```python
from build123d import *

# Parameters (mm, degrees)
EXTRUDE_1_DEPTH             = 5
SKETCH_2_R                  = 1.6
CUT_EXTRUDE_1_DEPTH         = 5
PATTERN_LINEAR_1_COUNT      = 2
PATTERN_LINEAR_1_PITCH      = 58
PATTERN_LINEAR_1_COUNT_DIR2 = 2
PATTERN_LINEAR_1_PITCH_DIR2 = 49
SKETCH_3_R                  = 2.6
CUT_EXTRUDE_2_DEPTH         = 10
PATTERN_LINEAR_2_COUNT      = 2
PATTERN_LINEAR_2_PITCH      = 33
PATTERN_LINEAR_2_COUNT_DIR2 = 2
PATTERN_LINEAR_2_PITCH_DIR2 = 33
SKETCH_4_R                  = 1.65
CUT_EXTRUDE_4_DEPTH         = 10


with BuildPart() as part:
    # Эскиз1 → Бобышка-Вытянуть1 (new body)
    with BuildSketch(Plane(origin=(0, 0, 0), x_dir=(1, 0, 0), z_dir=(0, 1, 0))):
        Polygon((0, 0), (170, 0), (170, 60), (110, 190), (60, 190), (0, 60), align=None)
    extrude(amount=EXTRUDE_1_DEPTH)

    # Эскиз2 → Вырез-Вытянуть1 (cut)
    with BuildSketch(Plane(origin=(0, 5, 0), x_dir=(1, 0, 0), z_dir=(0, 1, 0))):
        with Locations(Location((60.5, 20, 0), (0, 0, 270))):
            Circle(SKETCH_2_R)
    cut_extrude_1 = extrude(amount=-CUT_EXTRUDE_1_DEPTH, mode=Mode.SUBTRACT)

    # Линейный массив1: Cut-Extrude 1 2 × 2
    with Locations(*[(j * PATTERN_LINEAR_1_PITCH_DIR2, 0, -i * PATTERN_LINEAR_1_PITCH) for i in range(PATTERN_LINEAR_1_COUNT) for j in range(PATTERN_LINEAR_1_COUNT_DIR2) if (i, j) != (0, 0)]):
        add(cut_extrude_1, mode=Mode.SUBTRACT)

    # Эскиз3 → Вырез-Вытянуть2 (cut)
    with BuildSketch(Plane(origin=(0, 5, 0), x_dir=(1, 0, 0), z_dir=(0, 1, 0))):
        with Locations(Location((101.5, 180, 0), (0, 0, 270))):
            Circle(SKETCH_3_R)
    cut_extrude_2 = extrude(amount=-CUT_EXTRUDE_2_DEPTH, mode=Mode.SUBTRACT)

    # Линейный массив2: Cut-Extrude 2 2 × 2
    with Locations(*[(-i * PATTERN_LINEAR_2_PITCH, 0, j * PATTERN_LINEAR_2_PITCH_DIR2) for i in range(PATTERN_LINEAR_2_COUNT) for j in range(PATTERN_LINEAR_2_COUNT_DIR2) if (i, j) != (0, 0)]):
        add(cut_extrude_2, mode=Mode.SUBTRACT)

    # Эскиз4 → Вырез-Вытянуть4 (cut)
    with BuildSketch(Plane(origin=(0, 5, 0), x_dir=(1, 0, 0), z_dir=(0, 1, 0))):
        with Locations(Location((23.75, 8.999743724, 0), (0, 0, 270))):
            Circle(SKETCH_4_R)
        with Locations(Location((23.75, 20.999743724, 0), (0, 0, 270))):
            Circle(SKETCH_4_R)
        with Locations(Location((146.25, 20.999743724, 0), (0, 0, 270))):
            Circle(SKETCH_4_R)
        with Locations(Location((146.25, 8.999743724, 0), (0, 0, 270))):
            Circle(SKETCH_4_R)
        with Locations(Location((45.274277733, 101.419560045, 0), (0, 0, 270))):
            Circle(SKETCH_4_R)
        with Locations(Location((40.245579603, 90.524047431, 0), (0, 0, 270))):
            Circle(SKETCH_4_R)
        with Locations(Location((126.821084869, 96.879607741, 0), (0, 0, 270))):
            Circle(SKETCH_4_R)
        with Locations(Location((131.849782999, 85.984095127, 0), (0, 0, 270))):
            Circle(SKETCH_4_R)
    extrude(amount=-CUT_EXTRUDE_4_DEPTH, mode=Mode.SUBTRACT)


solid = part.part
```
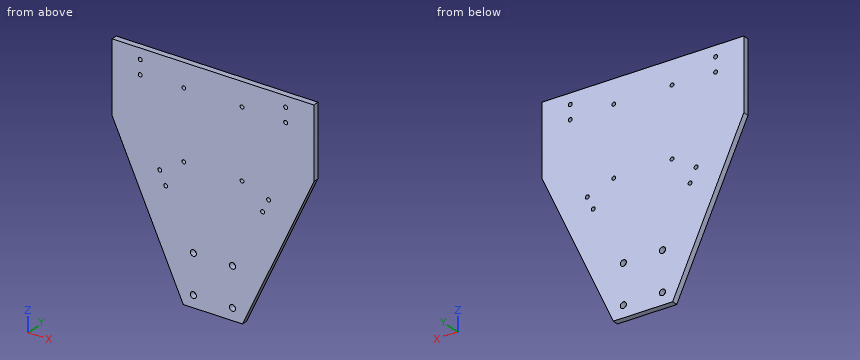
Geometry check sheet. Reference: the model listing, model coordinates, mm. Coordinates: 2 decimals unless noted, no trailing zeros. Order: outer loops, then holes, each group sorted by start corner. A loop starts at its lowest first (then second) coordinate and runs counter-clockwise, first axis right, second up. Notation, with made-up numbers: (59.25, 49) - (95.25, 49) arc R18 cw to (95.25, 82) - close; hole circle Ø5 at (72, 32.25). An arc over 180 degrees is marked (long way). Answer as a JSON object with one key per item and string values. Group by question number.
Item 1: Sectioned sample at B-B, the plane z = -180. Record the cut outline in (x, y), and give its area (3 significant figures).
Item 2: Sectioned sample at C-C, the plane y = 4.2. Give the number of separate pieces and of enclosed holes in the cut face, and give its area (3 significant figures).
Item 3: Sectioned sample at A-A, the plane x = 101.5. Record the cut outline in (y, z), and give its area (3 significant figures).
Item 4: Depth check by flat-ended pin: pin 1 Ø1 at (y, z) = (2, -162) entering from -X; pin 2 Ø1.5 at (y, z) = (3.5, -141) entering from -X. Enter the tip coordinate at first touch or a pass-through.
Item 5: Sectioned sample at D-D, the plane x = 12. Record the cut outline in (y, z), and give its area (3 significant figures).
Item 6: Scan lines: probe 1 along Z at (x, y) = (109.5, 3.2); probe 2 along X at (y, z) = (1.2, -147); probe 3 along Z at (x, y) = (70, 1.3). Record each from-to range of solid material in increasing order.
Resolved:
{
 "1": {"outline": "(55.38, 0) - (65.9, 0) - (65.9, 5) - (55.38, 5) - close; (71.1, 0) - (98.9, 0) - (98.9, 5) - (71.1, 5) - close; (104.1, 0) - (114.62, 0) - (114.62, 5) - (104.1, 5) - close", "area": "244 mm^2"},
 "2": {"separate pieces": "1", "enclosed holes": "16", "area": "24,300 mm^2"},
 "3": {"outline": "(0, -190) - (5, -190) - (5, -182.6) - (0, -182.6) - close; (0, -177.4) - (5, -177.4) - (5, -149.6) - (0, -149.6) - close; (0, -144.4) - (5, -144.4) - (5, 0) - (0, 0) - close", "area": "898 mm^2"},
 "4": {"pin 1": "x = 46.85", "pin 2": "x = 37.04"},
 "5": {"outline": "(0, -86) - (5, -86) - (5, 0) - (0, 0) - close", "area": "430 mm^2"},
 "6": {"probe 1": "-190 to -79.6, -76.4 to -21.6, -18.4 to 0", "probe 2": "40.15 to 65.9, 71.1 to 98.9, 104.1 to 129.85", "probe 3": "-190 to -182.12, -177.88 to -149.12, -144.88 to 0"}
}
